Geometry: final body of the model. Coordinates: model frame, mm. Face numbers are marked on the shaded views. A direction names the side the tool comes from. Give positions to 0.01 mm unless a question says otherwise; leave off trailing zeros. Order: outer loops, then holes, each group sorted by start corner. A loop starts at its lowest first (then second) coordinate and runs counter-clockwise, first axis right, second up. Notation, with made-up numbers: (-33.5, -21) - (20.5, -21) arc R28 ccw to (20.5, 18) - close; hole circle Ø2 at (6, 11.25). An arc over 180 degrees is marked (long way). Use one line per item in the form item = value.
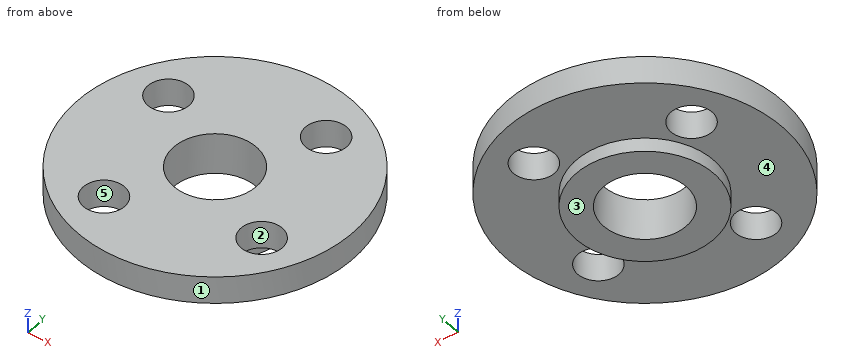
from build123d import *

# Parameters (mm, degrees)
SKETCH_1_R          = 5
SKETCH_1_R_2        = 3
EXTRUDE_1_DEPTH     = 1
SKETCH_2_R          = 10
SKETCH_2_R_2        = 3
EXTRUDE_2_DEPTH     = 2
SKETCH_3_R          = 1.5
CUT_EXTRUDE_1_DEPTH = 15.456832295


with BuildPart() as part:
    # 草图1 → 凸台-拉伸1 (new body)
    with BuildSketch(Plane.XY):
        Circle(SKETCH_1_R)
        Circle(SKETCH_1_R_2, mode=Mode.SUBTRACT)
    extrude(amount=EXTRUDE_1_DEPTH)

    # 草图2 → 凸台-拉伸2 (add)
    with BuildSketch(Plane.XY.offset(1)):
        Circle(SKETCH_2_R)
        Circle(SKETCH_2_R_2, mode=Mode.SUBTRACT)
    extrude(amount=EXTRUDE_2_DEPTH)

    # 草图3 → 切除-拉伸1 (cut, through all)
    with BuildSketch(Plane.XY.offset(3)):
        with Locations((3.427604113, 6.103403153)):
            Circle(SKETCH_3_R)
        with Locations((6.103403153, -3.427604113)):
            Circle(SKETCH_3_R)
        with Locations((-3.427604113, -6.103403153)):
            Circle(SKETCH_3_R)
        with Locations((-6.103403153, 3.427604113)):
            Circle(SKETCH_3_R)
    extrude(amount=-CUT_EXTRUDE_1_DEPTH, mode=Mode.SUBTRACT)


solid = part.part
(1) Cut plane B-B on y = -2.5. Output: boundary loops of the cut face in (x, z).
Computed values:
outline = (-9.68, 1) - (-4.33, 1) - (-4.33, 0) - (-1.66, 0) - (-1.66, 3) - (-9.68, 3) - close; (1.66, 0) - (4.33, 0) - (4.33, 1) - (4.92, 1) - (4.92, 3) - (1.66, 3) - close; (7.28, 1) - (9.68, 1) - (9.68, 3) - (7.28, 3) - close
(2) Contact query for flat-ended pins moving along their axis: pin 1 Ø2.5 at (x, y) = (3.43, 6.1) entering from +Z; pin 2 Ø10 at (x, y) = (-1.5, 5) entering from -Z; pin 3 Ø3.5 at (x, y) = (-3.43, -6.1) entering from -Z. Output: stop coordinate, or through.
Computed values:
pin_1 = through
pin_2 = 0
pin_3 = 1
(3) Cut plane A-A on x = 0. Output: boundary loops of the cut face in (y, z), plus the area to 3 significant figures.
Computed values:
outline = (-10, 1) - (-5, 1) - (-5, 0) - (-3, 0) - (-3, 3) - (-10, 3) - close; (3, 0) - (5, 0) - (5, 1) - (10, 1) - (10, 3) - (3, 3) - close
area = 32.0 mm²
(4) Pull-direction query (X, two-part tool) for the marked faces 1, 2 and 3; classes: released by +X, released by -X, zero draft, split by the parting line, or undercut.
Computed values:
face_1 = split by the parting line
face_2 = undercut
face_3 = zero draft
(5) Reachability of the marked faces 4 and 5 from +Z, -Z, +X, -X, +Y, -Y: full face, straight path, thin tool, end or side. Return the list, or none.
Computed values:
face_4 = -Z
face_5 = +Z, -Z
(6) Cut plane D-D on z = 2.4. Output: boundary loops of the cut face in (x, y), plus the area to 3 significant figures.
Computed values:
outline = circle Ø20 at (0, 0); hole circle Ø3 at (-6.1, 3.43); hole circle Ø3 at (-3.43, -6.1); hole circle Ø6 at (0, 0); hole circle Ø3 at (3.43, 6.1); hole circle Ø3 at (6.1, -3.43)
area = 258 mm²
(7) Ray query, line 1 along Y through (x, z) = (-4.75, 1.65); line 2 along X through (y, z) = (-2.75, 2.4); line 3 along Z through (x, y) = (-6.5, 6). Return the intervals inside material, ascending.
Computed values:
line_1 = -8.8 to -6.81, -5.4 to 2.78, 4.07 to 8.8
line_2 = -9.61 to -1.2, 1.2 to 4.77, 7.44 to 9.61
line_3 = 1 to 3
